from build123d import *

# Parameters (mm, degrees)
ESQUISSE2_R        = 2
ESQUISSE2_2_R      = 2
BOSS_EXTRU_1_DEPTH = 30


with BuildPart() as part:
    # Balayage1: sweep along a path in Esquisse1
    with BuildLine(Plane.XY) as balayage1_path:
        Line((0, 0), (12.816178594, 0))
        ThreePointArc((12.816178594, 0), (14.868299454, 0.361844275), (16.672904253, 1.403733341))
        Line((16.672904253, 1.403733341), (59.940468109, 37.709530215))
        ThreePointArc((59.940468109, 37.709530215), (63.014036614, 39.061932725), (66.332903338, 38.551110279))
        Line((66.332903338, 38.551110279), (111.436464109, 17.518974481))
    # Esquisse2 → Balayage1 (sweep)
    with BuildSketch(Plane(origin=(0, 0, 0), x_dir=(0, 0, -1), z_dir=(1, 0, 0))):
        with Locations((0, 2)):
            Circle(ESQUISSE2_R)
    sweep(path=balayage1_path.line)

    # Esquisse2<2> → Boss.-Extru.1 (add)
    with BuildSketch(Plane(origin=(0, 0, 0), x_dir=(0, 0, -1), z_dir=(1, 0, 0))):
        with Locations((0, 2)):
            Circle(ESQUISSE2_2_R)
    extrude(amount=-BOSS_EXTRU_1_DEPTH)


solid = part.part
Design review of the part built by this model. Coordinates are the model's own, in mm. Coordinates: 2 decimals unless noted, no trailing zeros. Order: outer loops, then holes, each group sorted by start corner. A loop starts at its lowest first (then second) coordinate and runs counter-clockwise, first axis right, second up. Notation, with made-up numbers: (25.25, 53) -> (61.25, 53) arc R24 ccw to (61.25, 68) -> close; hole circle Ø6 at (32.25, 57.5). An arc over 180 degrees is marked (long way). One line per item, written item: value.
1) Draft analysis for pull direction X (two halves, no side actions). For faces 1 (the face through (90.88, 31.5, 0.26)), 2 (the face through (-8, 0, 0)), 3 (the face through (-30, 2, 0)), state which applies: +X half, -X half, draft (parallel to the pull), parting line (faces both ways), or undercut.
Output values:
face 1: undercut
face 2: draft
face 3: -X half
2) Clearance check with a flat-ended pin moving along its axis: P1, Ø1.5, axis at x = 28, z = -0.5, coming from the -Y side. State where the tip first meets the part, or that it passes through.
Output values:
P1: stops at y = 10.33
3) To check wall thickness, follow probe 1 along Y at (x, z) = (11, 0.2); probe 2 along X at (y, z) = (25.5, 1.2); probe 3 along X at (y, z) = (28, 1.1). State the ranges of each line that lie inside material, in increasing order. Write a range as [from, to].
Output values:
probe 1: y = [0.01, 3.99]
probe 2: x = [39.79, 44.77], [95.27, 102.84]
probe 3: x = [42.66, 47.86], [89.74, 97.64]
4) We need section A-A, the plane z = -0.05. Give the boundary of the cut face in (x, y), then the cut area to 3 significant figures.
Output values:
outline: (-30, 0) -> (12.82, 0) arc R6 ccw to (16.67, 1.4) -> (59.94, 37.71) arc R6 cw to (66.33, 38.55) -> (111.44, 17.52) -> (113.13, 21.14) -> (68.02, 42.18) arc R10 ccw to (57.37, 40.77) -> (14.1, 4.47) arc R2 cw to (12.82, 4) -> (-30, 4) -> close
area: 644 mm2
5) We need section B-B, the plane x = -4.5. Give the boundary of the cut face in (y, z), then the cut area to 3 significant figures.
Output values:
outline: circle Ø4 at (2, 0)
area: 12.6 mm2
